Part model, mm, in its own coordinate system. A direction names the side the tool comes from. Give positions to 0.01 mm unless a question says otherwise; leave off trailing zeros. Write each loop counter-clockwise with the first axis right and the second up, starting at its lowest first coordinate (ties: lowest second). Pieces come first, ordered by that corner, then holes.
from build123d import *

# Parameters (mm, degrees)
SKETCH1_R                       = 28.5
BOSS_EXTRUDE1_DEPTH             = 15
FILLET1_R                       = 7.5
F_32_0_116_DIAMETER_HOLE4_D     = 2.9464
F_32_0_116_DIAMETER_HOLE4_DEPTH = 3
F_32_0_116_DIAMETER_HOLE4_TIP   = 0.885187864


with BuildPart() as part:
    # Sketch1 → Boss-Extrude1 (new body)
    with BuildSketch(Plane(origin=(0, 0, 0), x_dir=(1, 0, 0), z_dir=(0, 1, 0))):
        with Locations(Location((0, 0, 0), (0, 0, 270))):
            Circle(SKETCH1_R)
    extrude(amount=BOSS_EXTRUDE1_DEPTH)

    # Fillet1
    fillet1_edges = [part.edges().sort_by_distance(p)[0] for p in [
        (0, 15, -28.5),
    ]]
    fillet(fillet1_edges, radius=FILLET1_R)

    # #32 (0.116) Diameter Hole4
    with Locations(Plane(origin=(0, 0, 0), x_dir=(-1, 0, 0), z_dir=(0, -1, 0))):
        with Locations((-16.25, 16.25), (16.25, 16.25), (16.25, -16.25), (-16.25, -16.25)):
            Hole(F_32_0_116_DIAMETER_HOLE4_D / 2, depth=F_32_0_116_DIAMETER_HOLE4_DEPTH)
            with Locations((0, 0, -(F_32_0_116_DIAMETER_HOLE4_DEPTH + F_32_0_116_DIAMETER_HOLE4_TIP / 2))):  # 118° drill point
                Cone(0, F_32_0_116_DIAMETER_HOLE4_D / 2, F_32_0_116_DIAMETER_HOLE4_TIP, mode=Mode.SUBTRACT)


solid = part.part
1) 3-axis set-ups, long thin cutter, end or side, ignore diameter. For faces 1 (the cylindrical face through (-14.889, 1.521, 16.814)), 2 (the flat face through (0, 0, 0)): which of +Z, -Z, +X, -X, +Y, -Y reach the whole face in a straight line?
Check result:
face 1: -Y
face 2: +Z, -Z, +X, -X, -Y
2) Saw through at B-B (z = 0). Write the cut outline in (x, y).
Check result:
outline: (-28.5, 0) - (28.5, 0) - (28.5, 7.5) arc R7.5 ccw to (21, 15) - (-21, 15) arc R7.5 ccw to (-28.5, 7.5) - close
3) Saw through at D-D (y = 6). Write the cut outline in (x, z).
Check result:
outline: circle Ø57 at (0, 0)
4) Mould opens along Z. For faces 3 (the flat face through (0, 15, 0)), 4 (the conical face through (16.006, 3.731, 16.173)), 5 (the cylindrical face through (-27.82, 3.7, -6.18)) say: +Z half, -Z half, draft (parallel to the pull), parting line (faces both ways), or undercut.
Check result:
face 3: draft
face 4: undercut
face 5: parting line
5) Drill centre lines: L1, parallel to X at y = 2.35, z = -16.25; L2, parallel to Y at x = -21, z = -2. Where is each one in solid material? Low to high.
Check result:
L1: x = -23.41 to -17.72, -14.78 to 14.78, 17.72 to 23.41
L2: y = 0 to 15
6) Saw through at A-A (y = 1.25). Write the cut outline in (x, z), and give its area (3 significant figures).
Check result:
outline: circle Ø57 at (0, 0); hole circle Ø2.95 at (-16.25, -16.25); hole circle Ø2.95 at (-16.25, 16.25); hole circle Ø2.95 at (16.25, -16.25); hole circle Ø2.95 at (16.25, 16.25)
area: 2,520 mm2
7) Saw through at C-C (x = 0). Write the cut outline in (y, z).
Check result:
outline: (0, -28.5) - (7.5, -28.5) arc R7.5 ccw to (15, -21) - (15, 21) arc R7.5 ccw to (7.5, 28.5) - (0, 28.5) - close
8) Flat gauge pins, fed straight in: P1, Ø3, axis at y = 5, z = 10, coming from the -X side; P2, Ø2.5, axis at x = 16.25, z = 16.25, coming from the -Y side; P3, Ø4, axis at x = -16.25, z = 16.25, coming from the -Y side; P4, Ø4, axis at x = 16, z = -21.5, coming from the +Y side. Where does each tip first touch, or does it go through?
Check result:
P1: stops at x = -27.2
P2: stops at y = 3.13
P3: stops at y = 0
P4: stops at y = 13.97
